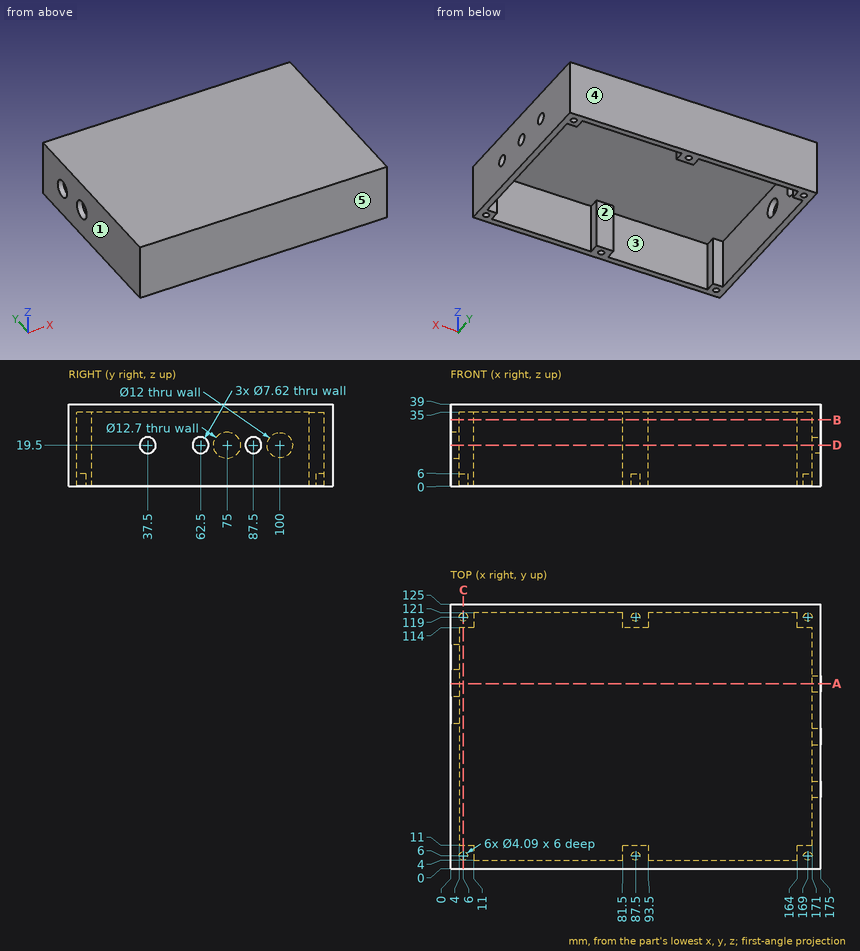
Verification items for this drawing (mm, ordinates from the low corner). A direction names the side the tool comes from. Give positions to 0.01 mm unless a question says otherwise; leave off trailing zeros. Loops run counter-clockwise (first coordinate to the right, second up) from the corner with the lowest first, then second, coordinate; pieces in that order, holes last.
(1) Section check D-D on z = 19.5. Count the separate pieces of the cut face and the enclosed holes in it, then the cut area to 3 significant figures.
From the geometry:
separate pieces: 5
enclosed holes: 0
area: 2,510 mm2
(2) Section check A-A on y = 87.5. Record the cut outline in (x, z), then the cut area to 3 significant figures.
From the geometry:
outline: (0, 0) - (4, 0) - (4, 35) - (171, 35) - (171, 23.31) - (175, 23.31) - (175, 39) - (0, 39) - close; (171, 0) - (175, 0) - (175, 15.69) - (171, 15.69) - close
area: 950 mm2
(3) Depth check by flat-ended pin: pin 1 Ø2.5 at (x, y) = (87.5, 119) entering from -Z; pin 2 Ø6 at (x, y) = (95.5, 72) entering from -Z. Enter the tip coordinate at first touch or a pass-through.
From the geometry:
pin 1: stops at z = 6
pin 2: stops at z = 35
(4) Set-up check for the marked faces 1 and 2: record each of +Z, -Z, +X, -X, +Y, -Y from which the full face is reachable in a straight line by a thin tool's end or side.
From the geometry:
face 1: +Z, -Z, -X, +Y, -Y
face 2: -Z
(5) Release check for a two-part mould opening along Y. For the marked faces 3, 4 and 5 record: released by +Y, released by -Y, zero draft, split by the parting line, or undercut.
From the geometry:
face 3: undercut
face 4: released by +Y
face 5: released by -Y
(6) Thickness scan on L1, parallel to Y at x = 6, z = 2 (3 decimals); L2, parallel to X at y = 10, z = 26.5; L3, parallel to Y at x = 115.5, z = 2.5. Record the ranges inside material, lowest first.
From the geometry:
L1: y = 0 to 3.955, 8.045 to 11, 114 to 116.955, 121.045 to 125
L2: x = 0 to 11, 81.5 to 93.5, 164 to 175
L3: y = 0 to 4, 121 to 125
(7) Section check B-B on z = 31.5. Record the cut outline in (x, y).
From the geometry:
outline: (0, 0) - (175, 0) - (175, 125) - (0, 125) - close; hole (4, 11) - (11, 11) - (11, 4) - (81.5, 4) - (81.5, 11) - (93.5, 11) - (93.5, 4) - (164, 4) - (164, 11) - (171, 11) - (171, 114) - (164, 114) - (164, 121) - (93.5, 121) - (93.5, 114) - (81.5, 114) - (81.5, 121) - (11, 121) - (11, 114) - (4, 114) - close
(8) Section check C-C on x = 6. Record the cut outline in (y, z) (3 decimals), then the cut area to 3 significant figures.
From the geometry:
outline: (0, 0) - (3.955, 0) - (3.955, 6) - (8.045, 6) - (8.045, 0) - (11, 0) - (11, 35) - (114, 35) - (114, 0) - (116.955, 0) - (116.955, 6) - (121.045, 6) - (121.045, 0) - (125, 0) - (125, 39) - (0, 39) - close
area: 1,220 mm2
